Verification items for the finished model (mm, model axes). Round coordinates to 2 decimals unless told otherwise and drop trailing zeros. Order: outer loops, then holes, each group sorted by start corner. A loop starts at its lowest first (then second) coordinate and runs counter-clockwise, first axis right, second up.
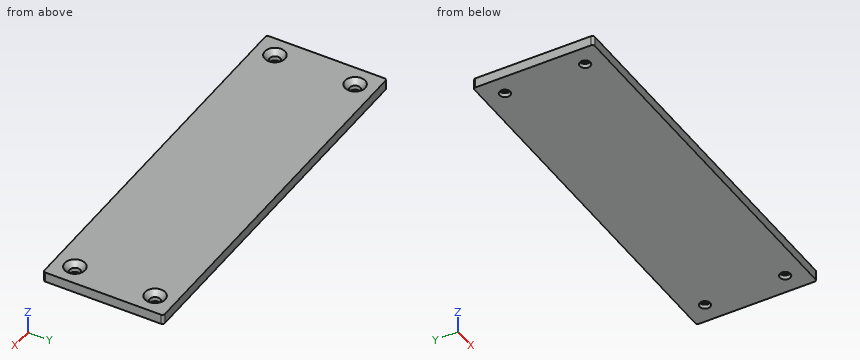
```python
from build123d import *

# Parameters (mm, degrees)
SKETCH1_W                                   = 241.3
SKETCH1_H                                   = 76.2
BOSS_EXTRUDE1_DEPTH                         = 6.35
CSK_FOR_1_4_FLAT_HEAD_MACHINE_SCREW_2_COUNT = 2
CSK_FOR_1_4_FLAT_HEAD_MACHINE_SCREW_2_PITCH = 50.8
CSK_FOR_1_4_FLAT_HEAD_MACHINE_SCREW_3_COUNT = 2
CSK_FOR_1_4_FLAT_HEAD_MACHINE_SCREW_3_PITCH = 215.9
CSK_FOR_1_4_FLAT_HEAD_MACHINE_SCREW_4_COUNT = 2
CSK_FOR_1_4_FLAT_HEAD_MACHINE_SCREW_4_PITCH = 221.795964796
FILLET1_R                                   = 1.5875


with BuildPart() as part:
    # Sketch1 → Boss-Extrude1 (new body)
    with BuildSketch(Plane.XY):
        Rectangle(SKETCH1_W, SKETCH1_H)
    extrude(amount=BOSS_EXTRUDE1_DEPTH)

    # Sketch4 → CSK for 1/4 Flat Head Machine Screw (100)1 (revolve, cut)
    with BuildSketch(Plane(origin=(107.95, 25.4, 6.35), x_dir=(0, -1, 0), z_dir=(1, 0, 0))):
        Polygon((0, 0), (0, 6.35), (3.3782, 6.35), (3.3782, 3.520932584), (6.4389, 0), align=None)
    csk_for_1_4_flat_head_machine_screw_100 = revolve(axis=Axis((107.95, 25.4, 12.7), (0, 0, -1)), mode=Mode.SUBTRACT)

    # CSK for 1_4 Flat Head Machine Screw  2: CSK for 1/4 Flat Head Machine Screw (100)1 ×2
    with Locations(*[(0, -i * CSK_FOR_1_4_FLAT_HEAD_MACHINE_SCREW_2_PITCH, 0) for i in range(1, CSK_FOR_1_4_FLAT_HEAD_MACHINE_SCREW_2_COUNT)]):
        add(csk_for_1_4_flat_head_machine_screw_100, mode=Mode.SUBTRACT)

    # CSK for 1_4 Flat Head Machine Screw  3: CSK for 1/4 Flat Head Machine Screw (100)1 ×2
    with Locations(*[(-i * CSK_FOR_1_4_FLAT_HEAD_MACHINE_SCREW_3_PITCH, 0, 0) for i in range(1, CSK_FOR_1_4_FLAT_HEAD_MACHINE_SCREW_3_COUNT)]):
        add(csk_for_1_4_flat_head_machine_screw_100, mode=Mode.SUBTRACT)

    # CSK for 1_4 Flat Head Machine Screw  4: CSK for 1/4 Flat Head Machine Screw (100)1 ×2
    with Locations(*[Vector(-0.973417168, -0.229039334, 0) * (i * CSK_FOR_1_4_FLAT_HEAD_MACHINE_SCREW_4_PITCH) for i in range(1, CSK_FOR_1_4_FLAT_HEAD_MACHINE_SCREW_4_COUNT)]):
        add(csk_for_1_4_flat_head_machine_screw_100, mode=Mode.SUBTRACT)

    # Fillet1
    fillet1_edges = [part.edges().sort_by_distance(p)[0] for p in [
        (120.65, -38.1, 3.175),
        (-120.65, -38.1, 3.175),
        (-120.65, 38.1, 3.175),
        (120.65, 38.1, 3.175),
    ]]
    fillet(fillet1_edges, radius=FILLET1_R)


solid = part.part
```
1) Sectioned sample at A-A on y = 25.4. Record the cut outline in (x, z).
2) Go/stop test with flat-tipped pins: pin 1 Ø4 at (x, y) = (-107.95, -25.4) entering from +Z; pin 2 Ø11 at (x, y) = (107.95, -25.4) entering from +Z. Record where each tip stops, or that it passes through.
3) Sectioned sample at B-B on x = -107.95. Record the cut outline in (y, z), then the cut area to 3 significant figures.
4) Scan lines: probe 1 along X at (y, z) = (-25.4, 1.2); probe 2 along Y at (x, z) = (107.95, 0.75); probe 3 along X at (y, z) = (-23.5, 0.75). Record each from-to range of solid material in increasing order.
Returned:
1. outline: (-120.65, 0) - (-111.33, 0) - (-111.33, 2.83) - (-114.39, 6.35) - (-120.65, 6.35) - close; (-104.57, 0) - (104.57, 0) - (104.57, 2.83) - (101.51, 6.35) - (-101.51, 6.35) - (-104.57, 2.83) - close; (111.33, 0) - (120.65, 0) - (120.65, 6.35) - (114.39, 6.35) - (111.33, 2.83) - close
2. pin 1: passes through
2. pin 2: stops at z = 5.27
3. outline: (-38.1, 0) - (-28.78, 0) - (-28.78, 2.83) - (-31.84, 6.35) - (-38.1, 6.35) - close; (-22.02, 0) - (22.02, 0) - (22.02, 2.83) - (18.96, 6.35) - (-18.96, 6.35) - (-22.02, 2.83) - close; (28.78, 0) - (38.1, 0) - (38.1, 6.35) - (31.84, 6.35) - (28.78, 2.83) - close
3. area: 377 mm2
4. probe 1: x = -120.65 to -111.33, -104.57 to 104.57, 111.33 to 120.65
4. probe 2: y = -38.1 to -28.78, -22.02 to 22.02, 28.78 to 38.1
4. probe 3: x = -120.65 to -110.74, -105.16 to 105.16, 110.74 to 120.65
